Source: three-view drawing plus pictorial views. Frame: mm from the lowest corner of the part. A direction names the side the tool comes from. Give positions to 0.01 mm unless a question says otherwise; leave off trailing zeros. Loops run counter-clockwise (first coordinate to the right, second up) from the corner with the lowest first, then second, coordinate; pieces in that order, holes last. Notation, with made-up numbers: M 55,50.25 L 82,50.25 A14 cw 82,76.25 Z; hole C -34,-5.75 d7. An arc over 180 degrees is marked long. One line per item, written item: value. Start each with the question number.
(1) Pull-direction query (Y, two-part tool) for the marked faces 1, 2 and 3; classes: released by +Y, released by -Y, zero draft, split by the parting line, or undercut.
(2) Ray query, line 1 along Y through (x, z) = (17, 16.25); line 2 along X through (y, z) = (41.5, 2); line 3 along Y through (x, z) = (20.5, 1.25). Return the intervals inside material, ascending. Write a range as from..to.
(3) Pin query (flat end, axial travel): P1, Ø4, axis at y = 21.5, z = 2, coming from the -X side; P2, Ø12, axis at x = 21, y = 22, coming from the +Z side; P3, Ø2.5, axis at y = 33.5, z = 1.5, coming from the +X side. Return the tip coordinate at first contact, or that it passes through.
(4) Section D-D on x = 3. Output: boundary loops of the cut face in (y, z).
(5) Access query for the marked faces 4 and 5. Directions: +Z, -Z, +X, -X, +Y, -Y. A direction counts if a zero-diameter tool reaches every point of the face in a straight line with its end or side. Return the directions, or none.
(6) Section C-C on y = 25. Output: boundary loops of the cut face in (x, z).
(7) Section A-A on z = 17.5. Output: boundary loops of the cut face in (x, y), plus the area to 3 significant figures.
(8) Section B-B on x = 20. Output: boundary loops of the cut face in (y, z).
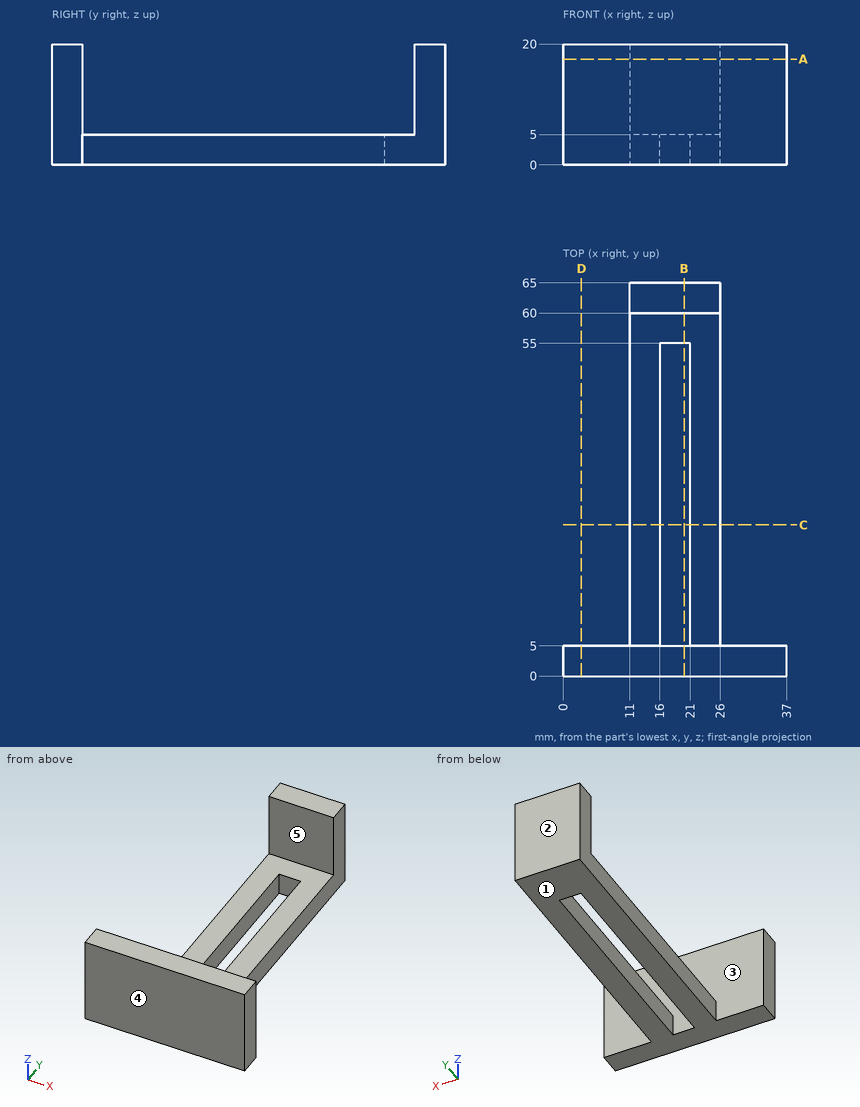
Output values:
1. face 1: zero draft
1. face 2: released by +Y
1. face 3: undercut
2. line 1: y = 0..5, 60..65
2. line 2: x = 11..16, 21..26
2. line 3: y = 0..5, 55..65
3. P1: stops at x = 11
3. P2: stops at z = 5
3. P3: stops at x = 26
4. outline: M 0,0 L 5,0 L 5,20 L 0,20 Z
5. face 4: +Z, -Z, +X, -X, -Y
5. face 5: +Z, +X, -X
6. outline: M 11,0 L 16,0 L 16,5 L 11,5 Z; M 21,0 L 26,0 L 26,5 L 21,5 Z
7. outline: M 0,0 L 37,0 L 37,5 L 0,5 Z; M 11,60 L 26,60 L 26,65 L 11,65 Z
7. area: 260 mm²
8. outline: M 0,0 L 5,0 L 5,20 L 0,20 Z; M 55,0 L 65,0 L 65,20 L 60,20 L 60,5 L 55,5 Z
